Input: part model. Units: mm. Frame: model coordinates. A direction names the side the tool comes from. Round coordinates to 2 decimals unless told otherwise and drop trailing zeros. Write each loop counter-clockwise with the first axis right and the second up, starting at its lowest first coordinate (ties: lowest second). Pieces come first, ordered by that corner, then holes. Notation, with made-up numbers: (80, 25.5) -> (114, 25.5) arc R26 cw to (114, 47.5) -> close; hole circle Ø2 at (13.25, 85.25). An arc over 180 degrees is marked (long way). Use CSV: the item, a comma, the result in double quotes.
```python
from build123d import *

# Parameters (mm, degrees)
SKETCH1_W           = 234
SKETCH1_H           = 75
BOSS_EXTRUDE1_DEPTH = 5.7
SKETCH2_W           = 5.7
SKETCH2_H           = 55
CUT_EXTRUDE1_DEPTH  = 5.7
SKETCH3_W           = 194
SKETCH3_H           = 12
SKETCH3_W_2         = 38.3
SKETCH3_H_2         = 10
CUT_EXTRUDE2_DEPTH  = 5.7
SKETCH4_W           = 174
SKETCH4_H           = 5.7
CUT_EXTRUDE3_DEPTH  = 5.7
SKETCH6_R           = 1.5
CUT_EXTRUDE4_DEPTH  = 3
SKETCH7_R           = 1.5
CUT_EXTRUDE5_DEPTH  = 3


with BuildPart() as part:
    # Sketch1 → Boss-Extrude1 (new body)
    with BuildSketch(Plane(origin=(0, 0, 0), x_dir=(1, 0, 0), z_dir=(0, 1, 0))):
        with Locations((117, 37.5)):
            Rectangle(SKETCH1_W, SKETCH1_H)
    extrude(amount=BOSS_EXTRUDE1_DEPTH)

    # Sketch2 → Cut-Extrude1 (cut)
    with BuildSketch(Plane(origin=(0, 5.7, 0), x_dir=(1, 0, 0), z_dir=(0, 1, 0))):
        with Locations((2.85, 37.5)):
            Rectangle(SKETCH2_W, SKETCH2_H)
        with Locations((231.15, 37.5)):
            Rectangle(SKETCH2_W, SKETCH2_H)
    extrude(amount=-CUT_EXTRUDE1_DEPTH, mode=Mode.SUBTRACT)

    # Sketch3 → Cut-Extrude2 (cut)
    with BuildSketch(Plane(origin=(0, 5.7, 0), x_dir=(1, 0, 0), z_dir=(0, 1, 0))):
        with Locations((117, 57)):
            Rectangle(SKETCH3_W, SKETCH3_H)
        with Locations((117, 32)):
            Rectangle(SKETCH3_W_2, SKETCH3_H_2)
        with BuildLine():
            Line((92.85, 27), (71.85, 27))
            ThreePointArc((71.85, 27), (69.021572875, 28.171572875), (67.85, 31))
            Line((67.85, 31), (67.85, 33))
            ThreePointArc((67.85, 33), (69.021572875, 35.828427125), (71.85, 37))
            Line((71.85, 37), (92.85, 37))
            Line((92.85, 37), (92.85, 27))
        make_face()
        with BuildLine():
            Line((162.15, 27), (141.15, 27))
            Line((141.15, 27), (141.15, 37))
            Line((141.15, 37), (162.15, 37))
            ThreePointArc((162.15, 37), (164.978427125, 35.828427125), (166.15, 33))
            Line((166.15, 33), (166.15, 31))
            ThreePointArc((166.15, 31), (164.978427125, 28.171572875), (162.15, 27))
        make_face()
    extrude(amount=-CUT_EXTRUDE2_DEPTH, mode=Mode.SUBTRACT)

    # Sketch4 → Cut-Extrude3 (cut)
    with BuildSketch(Plane(origin=(0, 5.7, 0), x_dir=(1, 0, 0), z_dir=(0, 1, 0))):
        with Locations((117, 72.15)):
            Rectangle(SKETCH4_W, SKETCH4_H)
    extrude(amount=-CUT_EXTRUDE3_DEPTH, mode=Mode.SUBTRACT)

    # Sketch6 → Cut-Extrude4 (cut)
    with BuildSketch(Plane.XZ):
        with Locations(Location((152, -66, 0), (0, 0, 270))):
            Circle(SKETCH6_R)
        with Locations(Location((82, -66, 0), (0, 0, 270))):
            Circle(SKETCH6_R)
        with Locations(Location((82, -43.5, 0), (0, 0, 270))):
            Circle(SKETCH6_R)
        with Locations(Location((152, -43.5, 0), (0, 0, 270))):
            Circle(SKETCH6_R)
    extrude(amount=-CUT_EXTRUDE4_DEPTH, mode=Mode.SUBTRACT)

    # Sketch7 → Cut-Extrude5 (cut)
    with BuildSketch(Plane.XZ):
        with Locations(Location((205, -66, 0), (0, 0, 270))):
            Circle(SKETCH7_R)
        with Locations(Location((160, -66, 0), (0, 0, 270))):
            Circle(SKETCH7_R)
        with Locations(Location((160, -46, 0), (0, 0, 270))):
            Circle(SKETCH7_R)
        with Locations(Location((205, -46, 0), (0, 0, 270))):
            Circle(SKETCH7_R)
        with Locations(Location((74, -66, 0), (0, 0, 270))):
            Circle(SKETCH7_R)
        with Locations(Location((29, -66, 0), (0, 0, 270))):
            Circle(SKETCH7_R)
        with Locations(Location((29, -46, 0), (0, 0, 270))):
            Circle(SKETCH7_R)
        with Locations(Location((74, -46, 0), (0, 0, 270))):
            Circle(SKETCH7_R)
    extrude(amount=-CUT_EXTRUDE5_DEPTH, mode=Mode.SUBTRACT)


solid = part.part
```
Item 1: First-contact query: pin 1 Ø0.9 at (x, z) = (152, -43.5) entering from -Y; pin 2 Ø3 at (x, y) = (123, 3) entering from -Z; pin 3 Ø3 at (y, z) = (4, -54.5) entering from +X; pin 4 Ø4 at (x, z) = (78, -60.5) entering from -Y. Flat tips, straight axial feed; report the tip coordinate or a pass-through.
Worked answers:
pin 1,"stops at y = 3"
pin 2,"stops at z = -69.3"
pin 3,"stops at x = 228.3"
pin 4,"passes through"
Item 2: Line query: line 1 (Z direction, x = 148, y = 2.7); line 2 (X direction, y = 5.15, z = -31.5); line 3 (Z direction, x = 152, y = 2.3). Output: solid intervals per line, ascending.
Worked answers:
line 1,"z = -69.3 to -63, -51 to -37, -27 to 0"
line 2,"x = 5.7 to 67.85, 92.85 to 97.85, 136.15 to 141.15, 166.15 to 228.3"
line 3,"z = -69.3 to -67.5, -64.5 to -63, -51 to -45, -42 to -37, -27 to 0"
Item 3: Section query D-D on y = 3.9. Give the number of separate pieces and of enclosed holes in the cut face, plus the area to 3 significant figures.
Worked answers:
separate pieces,"1"
enclosed holes,"4"
area,"12,700 mm²"
Item 4: Section query A-A on z = -56. Return the cut outline in (x, y), plus the area to 3 significant figures.
Worked answers:
outline,"(5.7, 0) -> (20, 0) -> (20, 5.7) -> (5.7, 5.7) -> close; (214, 0) -> (228.3, 0) -> (228.3, 5.7) -> (214, 5.7) -> close"
area,"163 mm²"
Item 5: Pull-direction query (X, two-part tool) for faces 5 (the face through (3, 3, -65)), 6 (the face through (82, 3, -27)), 7 (the face through (234, 3, -5)); classes: +X half, -X half, draft (parallel to the pull), parting line (faces both ways), or undercut.
Worked answers:
face 5,"draft"
face 6,"undercut"
face 7,"+X half"
Item 6: Section query B-B on x = 181. Return the cut outline in (y, z).
Worked answers:
outline,"(0, -69.3) -> (5.7, -69.3) -> (5.7, -63) -> (0, -63) -> close; (0, -51) -> (5.7, -51) -> (5.7, 0) -> (0, 0) -> close"
Item 7: Section query C-C on x = 112. Return the cut outline in (y, z), plus the area to 3 significant figures.
Worked answers:
outline,"(0, -69.3) -> (5.7, -69.3) -> (5.7, -63) -> (0, -63) -> close; (0, -51) -> (5.7, -51) -> (5.7, -37) -> (0, -37) -> close; (0, -27) -> (5.7, -27) -> (5.7, 0) -> (0, 0) -> close"
area,"270 mm²"
Item 8: Set-up query: faces 1 (the face through (30, 3, -72)), 2 (the face through (117, 3, -37)), 3 (the face through (231, 3, -65)), 4 (the face through (5.7, 3, -37)). Return all of +Z, -Z, +X, -X, +Y, -Y with unobstructed straight access to the full face (end or side cutting, diameter ignored); none if empty.
Worked answers:
face 1,"-Z, +Y, -Y"
face 2,"+Y, -Y"
face 3,"+X, +Y, -Y"
face 4,"-X, +Y, -Y"
